Can you work these out from the model? Positions are in its coordinate system, mm. A direction names the side the tool comes from. Give positions to 0.01 mm unless a question says otherwise; leave off trailing zeros. Order: outer loops, then holes, each group sorted by start corner. A loop starts at its lowest first (then second) coordinate and runs counter-clockwise, first axis right, second up. Notation, with made-up numbers: (3, -33) - (55, -33) arc R21 ccw to (55, -19) - close; hole circle Ø4 at (-26.75, 73). An arc over 180 degrees is marked (long way). Answer as a JSON object with one key per item and string values.
```python
from build123d import *

# Parameters (mm, degrees)
F1_DEPTH = 7.62
F3_DEPTH = 7.62


with BuildPart() as f1:
    # F0 (on Top) → F1 (new body)
    with BuildSketch(Plane.XY):
        with BuildLine():
            ThreePointArc((48.371598, 23.222628), (45.605213, 29.067693), (39.653465, 31.5964))
            Line((39.653465, 31.5964), (-43.028224, 31.5964))
            ThreePointArc((-43.028224, 31.5964), (-46.746564, 28.170959), (-48.371598, 23.383585))
            Line((-48.371598, 23.383585), (-48.371598, 21.795344))
            Line((-48.371598, 21.795344), (-48.371598, -20.670423))
            Line((-48.371598, -20.670423), (-48.371598, -23.518627))
            ThreePointArc((-48.371598, -23.518627), (-45.597003, -28.942544), (-40.112998, -31.5964))
            Line((-40.112998, -31.5964), (-37.68485, -31.5964))
            Line((-37.68485, -31.5964), (39.372232, -31.5964))
            Line((39.372232, -31.5964), (39.65662, -31.5964))
            ThreePointArc((39.65662, -31.5964), (45.067462, -29.752844), (48.371598, -25.088232))
            Line((48.371598, -25.088232), (48.371598, -19.545501))
            Line((48.371598, -19.545501), (48.371598, 21.795344))
            Line((48.371598, 21.795344), (48.371598, 23.222628))
        make_face()
        with BuildLine():
            ThreePointArc((48.371598, 21.795344), (48.399642, 22.508986), (48.371598, 23.222628))
            Line((48.371598, 23.222628), (48.371598, 21.795344))
        make_face()
        with BuildLine():
            Line((-48.371598, 21.795344), (-48.371598, 23.383585))
            ThreePointArc((-48.371598, 23.383585), (-48.402453, 22.589464), (-48.371598, 21.795344))
        make_face()
        with BuildLine():
            ThreePointArc((48.371598, -25.088232), (48.795049, -22.316866), (48.371598, -19.545501))
            Line((48.371598, -19.545501), (48.371598, -25.088232))
        make_face()
        with BuildLine():
            Line((-48.371598, -23.518627), (-48.371598, -20.670423))
            ThreePointArc((-48.371598, -20.670423), (-48.478048, -22.094525), (-48.371598, -23.518627))
        make_face()
        with BuildLine():
            ThreePointArc((39.372232, -31.5964), (39.514426, -31.59749), (39.65662, -31.5964))
            Line((39.65662, -31.5964), (39.372232, -31.5964))
        make_face()
        with BuildLine():
            Line((-37.68485, -31.5964), (-40.112998, -31.5964))
            ThreePointArc((-40.112998, -31.5964), (-38.898924, -31.673649), (-37.68485, -31.5964))
        make_face()
    extrude(amount=F1_DEPTH)

    # F2 (on face) → F3 (cut)
    with BuildSketch(Plane.XY.offset(7.62)):
        Polygon((17.155044, 0), (-15.186432, 16.170738), (-15.186432, -16.170738), align=None)
    extrude(amount=-F3_DEPTH, mode=Mode.SUBTRACT)


solid = f1.part
```
Q1. I'm going to push flat-ended pins straight in: pin 1 Ø4 at (y, z) = (2, 5) entering from +X; pin 2 Ø1.5 at (y, z) = (-25, 2.5) entering from -X; pin 3 Ø1 at (y, z) = (24.5, 5) entering from -X. Where does each tip first touch, or does it pass through?
Recorded:
{"pin 1": "stops at x = 48.37", "pin 2": "stops at x = -48.23", "pin 3": "stops at x = -48.3"}
Q2. I need wall thicknesses on L1, parallel to Y at x = -25.5, z = 5.25; L2, parallel to X at y = 18.5, z = 4.5; L3, parallel to Y at x = -7, z = 7.25. Which ranges of each line are inside material? Lowest first, please.
Recorded:
{"L1": "y = -31.6 to 31.6", "L2": "x = -48.37 to 48.37", "L3": "y = -31.6 to -12.08, 12.08 to 31.6"}
Q3. If we section it at D-D, the plane y = 26: Please give me the cut outline in (x, z), then the cut area to 3 significant figures.
Recorded:
{"outline": "(-47.82, 0) - (47.7, 0) - (47.7, 7.62) - (-47.82, 7.62) - close", "area": "728 mm^2"}
Q4. If we section it at B-B, the plane z = 2.75: Please give me the cut outline in (x, y).
Recorded:
{"outline": "(-48.37, -23.52) arc R9.58 ccw to (-40.11, -31.6) arc R9.58 ccw to (-37.68, -31.6) - (39.37, -31.6) arc R9.28 ccw to (39.66, -31.6) arc R9.28 ccw to (48.37, -25.09) arc R9.28 ccw to (48.37, -19.55) - (48.37, 21.8) arc R9.09 ccw to (48.37, 23.22) arc R9.09 ccw to (39.65, 31.6) - (-43.03, 31.6) arc R10.23 ccw to (-48.37, 23.38) arc R10.23 ccw to (-48.37, 21.8) - (-48.37, -20.67) arc R9.58 ccw to start; hole (-15.19, -16.17) - (17.16, 0) - (-15.19, 16.17) - close"}
Q5. We'd pull the mould along X, two halves only. Please class faces 3 (the face through (1.211, 7.972, 3.863)), 4 (the face through (-38.916, -31.674, 3.757)), 5 (the face through (10, 7, 0)): released by +X, released by -X, zero draft, split by the parting line, or undercut.
Recorded:
{"face 3": "undercut", "face 4": "split by the parting line", "face 5": "zero draft"}
Q6. If we section it at C-C, the plane y = -10.5: Please give me the cut outline in (x, z).
Recorded:
{"outline": "(-48.37, 0) - (-15.19, 0) - (-15.19, 7.62) - (-48.37, 7.62) - close; (-3.84, 0) - (48.37, 0) - (48.37, 7.62) - (-3.84, 7.62) - close"}
Q7. Which directions (+Z, -Z, +X, -X, +Y, -Y) give clear straight access to the entire face, cutting with the end or side of a thin tool? Please do faces 1 (the face through (-15.186, 0, 4)), 2 (the face through (0, -31.596, 4)).
Recorded:
{"face 1": "+Z, -Z", "face 2": "+Z, -Z, +X, -Y"}
Q8. If we section it at A-A, the plane x = 15.5: Please give me the cut outline in (y, z), then the cut area to 3 significant figures.
Recorded:
{"outline": "(-31.6, 0) - (-0.83, 0) - (-0.83, 7.62) - (-31.6, 7.62) - close; (0.83, 0) - (31.6, 0) - (31.6, 7.62) - (0.83, 7.62) - close", "area": "469 mm^2"}
